from build123d import *

# Parameters (mm, degrees)
SKETCH1_W            = 78
SKETCH1_H            = 78
BOSS_EXTRUDE1_DEPTH  = 2
SKETCH2_W            = 30
SKETCH2_H            = 30
BOSS_EXTRUDE2_DEPTH  = 60
SKETCH3_W            = 26
SKETCH3_H            = 26
CUT_EXTRUDE1_DEPTH   = 62
SKETCH4_W            = 28
SKETCH4_H            = 2.5
CUT_EXTRUDE2_DEPTH   = 28
SKETCH5_W            = 26
SKETCH5_H            = 10
CUT_EXTRUDE3_DEPTH   = 2
SKETCH6_W            = 28
SKETCH6_H            = 2.5
CUT_EXTRUDE4_DEPTH   = 1
SKETCH7_W            = 28
SKETCH7_H            = 2.5
CUT_EXTRUDE5_DEPTH   = 1
SKETCH14_R           = 1.75
BOSS_EXTRUDE8_DEPTH  = 5
SKETCH15_R           = 1.75
BOSS_EXTRUDE9_DEPTH  = 5
SKETCH16_W           = 4
SKETCH16_H           = 5
BOSS_EXTRUDE10_DEPTH = 2
SKETCH17_W           = 2
SKETCH17_H           = 10
BOSS_EXTRUDE11_DEPTH = 5
SKETCH18_W           = 10
SKETCH18_H           = 2
BOSS_EXTRUDE12_DEPTH = 3


with BuildPart() as part:
    # Sketch1 → Boss-Extrude1 (new body)
    with BuildSketch(Plane(origin=(0, 0, 0), x_dir=(1, 0, 0), z_dir=(0, 1, 0))):
        Rectangle(SKETCH1_W, SKETCH1_H)
    extrude(amount=BOSS_EXTRUDE1_DEPTH)

    # Sketch2 → Boss-Extrude2 (add)
    with BuildSketch(Plane(origin=(0, 2, 0), x_dir=(1, 0, 0), z_dir=(0, 1, 0))):
        with Locations((24, 24)):
            Rectangle(SKETCH2_W, SKETCH2_H)
    extrude(amount=BOSS_EXTRUDE2_DEPTH)

    # Sketch3 → Cut-Extrude1 (cut)
    with BuildSketch(Plane(origin=(0, 62, 0), x_dir=(1, 0, 0), z_dir=(0, 1, 0))):
        with Locations((24, 24)):
            Rectangle(SKETCH3_W, SKETCH3_H)
    extrude(amount=-CUT_EXTRUDE1_DEPTH, mode=Mode.SUBTRACT)

    # Sketch4 → Cut-Extrude2 (cut)
    with BuildSketch(Plane.ZY.offset(-9)):
        with Locations((-23.934548619, 3.25)):
            Rectangle(SKETCH4_W, SKETCH4_H)
    extrude(amount=-CUT_EXTRUDE2_DEPTH, mode=Mode.SUBTRACT)

    # Sketch5 → Cut-Extrude3 (cut)
    with BuildSketch(Plane.XY.offset(-9)):
        with Locations((24, 9)):
            Rectangle(SKETCH5_W, SKETCH5_H)
    extrude(amount=-CUT_EXTRUDE3_DEPTH, mode=Mode.SUBTRACT)

    # Sketch6 → Cut-Extrude4 (cut)
    with BuildSketch(Plane.ZY.offset(-37)):
        with Locations((-23, 7.5)):
            Rectangle(SKETCH6_W, SKETCH6_H)
    extrude(amount=-CUT_EXTRUDE4_DEPTH, mode=Mode.SUBTRACT)

    # Sketch7 → Cut-Extrude5 (cut)
    with BuildSketch(Plane(origin=(11, 0, 0), x_dir=(0, 0, -1), z_dir=(1, 0, 0))):
        with Locations((23, 7.5)):
            Rectangle(SKETCH7_W, SKETCH7_H)
    extrude(amount=-CUT_EXTRUDE5_DEPTH, mode=Mode.SUBTRACT)

    # Sketch14 → Boss-Extrude8 (add)
    with BuildSketch(Plane(origin=(0, 2, 0), x_dir=(1, 0, 0), z_dir=(0, 1, 0))):
        with Locations((-3.25, -24.64)):
            Circle(SKETCH14_R)
    extrude(amount=BOSS_EXTRUDE8_DEPTH)

    # Sketch15 → Boss-Extrude9 (add)
    with BuildSketch(Plane(origin=(0, 2, 0), x_dir=(1, 0, 0), z_dir=(0, 1, 0))):
        with Locations((-24.64, -3.25)):
            Circle(SKETCH15_R)
    extrude(amount=BOSS_EXTRUDE9_DEPTH)

    # Sketch16 → Boss-Extrude10 (add)
    with BuildSketch(Plane(origin=(0, 2, 0), x_dir=(1, 0, 0), z_dir=(0, 1, 0))):
        with Locations((22, -22.14)):
            Rectangle(SKETCH16_W, SKETCH16_H)
        with Locations((22, -27.14)):
            Rectangle(SKETCH16_W, SKETCH16_H)
    extrude(amount=BOSS_EXTRUDE10_DEPTH)

    # Sketch17 → Boss-Extrude11 (add)
    with BuildSketch(Plane(origin=(0, 2, 0), x_dir=(1, 0, 0), z_dir=(0, 1, 0))):
        with Locations((25, -24.64)):
            Rectangle(SKETCH17_W, SKETCH17_H)
    extrude(amount=BOSS_EXTRUDE11_DEPTH)

    # Sketch18 → Boss-Extrude12 (add)
    with BuildSketch(Plane(origin=(0, 2, 0), x_dir=(1, 0, 0), z_dir=(0, 1, 0))):
        with Locations((-24.64, 25)):
            Rectangle(SKETCH18_W, SKETCH18_H)
    extrude(amount=BOSS_EXTRUDE12_DEPTH)


solid = part.part
Work out the finished part from the listing and answer in its coordinate system (mm). A direction names the side the tool comes from. Round coordinates to 2 decimals unless told otherwise and drop trailing zeros. Order: outer loops, then holes, each group sorted by start corner. A loop starts at its lowest first (then second) coordinate and runs counter-clockwise, first axis right, second up. Notation, with made-up numbers: M 4.25,19 L 22.25,19 A25 ccw 22.25,37 Z; hole C 5.5,71.5 d5. An arc over 180 degrees is marked long. Put each result on its own line as item: value. Start each with the question number.
Q1. Section C-C, the plane x = 34.5 is taken. Write down the section's boundary in (y, z).
Q2. Section A-A, the plane z = -33 is taken. Write down the section's boundary in (x, y), and give its area (3 significant figures).
Q3. A tool of negligible diameter and unlimited length cuts with its end or side. For faces 1 (the flat face through (24, 14, -10)), 2 (the flat face through (24, 3, 29.64)), 3 (the flat face through (24, 3, 19.64)), 4 (the flat face through (11, 1, -24)), from which of +Z, -Z, +X, -X, +Y, -Y can it reach the whole face along a straight path? Write none if from no direction.
Q4. Flat-ended cylindrical pins translate along their axes: pin 1 (4 mm diameter, centred on x = 22.5, y = 4.5, fed in from +Z); pin 2 (1.5 mm diameter, centred on y = 55, z = -16, fed in from -X); pin 3 (0.6 mm diameter, centred on x = -23, z = -25, fed in from +Y). Find the tip coordinate at first contact, or state that the pin passes through.
Q5. Section B-B, the plane y = 16.5 is taken. Write down the section's boundary in (x, z), and give its area (3 significant figures).
Q6. For a pull along X with two mould halves and no side action, classify faces 5 (the flat face through (39, 29, -20)), 6 (the flat face through (25, 7, 25)), 7 (the cylindrical face through (-23.023, 4.465, 3.92)), 8 (the flat face through (38, 8, -23)) as pulls with the +X half, pulls with the -X half, needs draft (parallel to the pull), parting line crosses it, or undercut.
Q7. Straight lines are drawn through the part: L1, parallel to Z at x = 25, y = 3; L2, parallel to Z at x = 28.5, y = 57.5; L3, parallel to Z at x = 17, y = 5. For each, find the intervals that lie inside material, in ascending order. Write a range as [from, to].
Q8. Section D-D, the plane x = -24.64 is taken. Write down the section's boundary in (y, z).
Findings below:
1. outline: M 0,-39 L 62,-39 L 62,-37 L 4.5,-37 L 4.5,-37.93 L 2,-37.93 L 2,-37 L 0,-37 Z; M 0,-11 L 2,-11 L 2,-9.93 L 4,-9.93 L 4,-9 L 2,-9 L 2,39 L 0,39 Z; M 14,-11 L 62,-11 L 62,-9 L 14,-9 Z
2. outline: M -39,0 L 11,0 L 11,2 L -39,2 Z; M 9,4.5 L 11,4.5 L 11,6.25 L 10,6.25 L 10,8.75 L 11,8.75 L 11,62 L 9,62 Z; M 37,0 L 39,0 L 39,62 L 37,62 L 37,8.75 L 38,8.75 L 38,6.25 L 37,6.25 Z
2. area: 334 mm^2
3. face 1: +Z
3. face 2: +Z, +X, -X, +Y
3. face 3: +X, -X, +Y
3. face 4: +Y, -Y
4. pin 1: stops at z = 29.64
4. pin 2: stops at x = 9
4. pin 3: stops at y = 5
5. outline: M 9,-39 L 39,-39 L 39,-9 L 9,-9 Z; hole M 11,-37 L 37,-37 L 37,-11 L 11,-11 Z
5. area: 224 mm^2
6. face 5: pulls with the +X half
6. face 6: needs draft
6. face 7: parting line crosses it
6. face 8: undercut
7. L1: z = [-39, -37.93], [-9.93, -9], [19.64, 29.64]
7. L2: z = [-39, -37], [-11, -9]
7. L3: z = [-39, -37]
8. outline: M 0,-39 L 2,-39 L 2,-26 L 5,-26 L 5,-24 L 2,-24 L 2,1.5 L 7,1.5 L 7,5 L 2,5 L 2,39 L 0,39 Z
